from build123d import *

# Parameters (mm, degrees)
SKETCH1_W           = 5
SKETCH1_H           = 54.5
SKETCH1_H_2         = 3
BOSS_EXTRUDE3_DEPTH = 3
SKETCH1_5_W         = 5
SKETCH1_5_H         = 3
BOSS_EXTRUDE4_DEPTH = 11
SKETCH3_W           = 5
SKETCH3_H           = 1
BOSS_EXTRUDE5_DEPTH = 1.5
BOSS_EXTRUDE5_TAPER = 10
BOSS_EXTRUDE6_DEPTH = 5
SKETCH34_W          = 3.5
SKETCH34_H          = 12
BOSS_EXTRUDE2_DEPTH = 12
CUT_EXTRUDE2_REACH  = 46.911
SKETCH4_R           = 2.75


with BuildPart() as part:
    # Sketch1 → Boss-Extrude3 (new body)
    with BuildSketch(Plane.XY):
        with Locations((-78.011372184, 0)):
            Rectangle(SKETCH1_W, SKETCH1_H)
        with Locations((-78.011372184, -28.75)):
            Rectangle(SKETCH1_W, SKETCH1_H_2)
        with Locations((-78.011372184, 28.75)):
            Rectangle(SKETCH1_W, SKETCH1_H_2)
    extrude(amount=BOSS_EXTRUDE3_DEPTH)

    # Sketch1<5> → Boss-Extrude4 (add)
    with BuildSketch(Plane.XY):
        with Locations((-78.011372184, -28.75)):
            Rectangle(SKETCH1_5_W, SKETCH1_5_H)
        with Locations((-78.011372184, 28.75)):
            Rectangle(SKETCH1_5_W, SKETCH1_5_H)
    extrude(amount=-BOSS_EXTRUDE4_DEPTH)

    # Sketch3 → Boss-Extrude5 (add)
    with BuildSketch(Plane(origin=(0, -27.25, 0), x_dir=(1, 0, 0), z_dir=(0, 1, 0))):
        with Locations((-78.011372184, 10.5)):
            Rectangle(SKETCH3_W, SKETCH3_H)
    boss_extrude5 = extrude(amount=BOSS_EXTRUDE5_DEPTH, taper=BOSS_EXTRUDE5_TAPER)

    # Mirror1: Boss-Extrude5 across plane
    add(boss_extrude5.mirror(Plane.ZX))

    # Sketch5 → Boss-Extrude6 (add)
    with BuildSketch(Plane(origin=(-75.511372184, 0, 0), x_dir=(0, 0, -1), z_dir=(1, 0, 0))):
        Polygon((-3, 9.5), (-2, 9.5), (-2, -9.5), (-3, -9.5), (-3, -3.05), (-5.4, -3.05), (-5.4, -5.45), (-6.4, -5.45), (-8, -3.05), (-8, 3.05), (-6.4, 5.45), (-5.4, 5.45), (-5.4, 3.05), (-3, 3.05), align=None)
    extrude(amount=-BOSS_EXTRUDE6_DEPTH)

    # Sketch34 → Boss-Extrude2 (add)
    with BuildSketch(Plane(origin=(-75.511372184, -10.701352109, -2.52337685), x_dir=(0, 0, -1), z_dir=(1, 0, 0))):
        with Locations((-3.77337685, 10.701352109)):
            Rectangle(SKETCH34_W, SKETCH34_H)
    extrude(amount=BOSS_EXTRUDE2_DEPTH)

    # Sketch4 → Cut-Extrude2 (cut, up to next)
    with BuildSketch(Plane(origin=(-75.511372184, -10.701352109, 3), x_dir=(1, 0, 0), z_dir=(0, 0, 1)), mode=Mode.PRIVATE) as cut_extrude2_sk1:
        with Locations((6, 10.701352109)):
            Circle(SKETCH4_R)
    cut_extrude2_tool1 = extrude(cut_extrude2_sk1.sketch, amount=-CUT_EXTRUDE2_REACH, mode=Mode.PRIVATE) & part.part
    add(cut_extrude2_tool1.solids().sort_by_distance((-69.511372, 0, 3))[0], mode=Mode.SUBTRACT)


solid = part.part
The model under review builds one solid part; all positions refer to its coordinate system, in mm. A direction names the side the tool comes from. Coordinates: 2 decimals unless noted, no trailing zeros. Loops run counter-clockwise (first coordinate to the right, second up) from the corner with the lowest first, then second, coordinate; pieces in that order, holes last. Notation, with made-up numbers: (-13, -28) -> (41, -28) arc R9 cw to (41, -19) -> close; hole circle Ø5 at (15, 51.25). An arc over 180 degrees is marked (long way). Use a Markdown table: item, result. Add a question column.
1. Clearance check with flat-ended pins moving along their axes: pin 1 Ø8 at (x, z) = (-68, 0) entering from -Y; pin 2 Ø1.5 at (y, z) = (19.5, 3) entering from +X; pin 3 Ø0.7 at (x, z) = (-77, 4) entering from +Y. State where each tip first meets the part, or that it passes through.
2. Machinability: for faces 1 (the face through (-75.511, 19.9, 0.2)), 2 (the face through (-70, -6, 1)), 3 (the face through (-78, -27.25, -5)), 4 (the face through (-75.511, 0, 6)), which of the approach directions +Z, -Z, +X, -X, +Y, -Y give a long, thin tool a straight path to every point of the face, cutting with its end or side? Answer none if there is none.
3. Add section A-A on y = 0. Write out the cut boundary in (x, z).
4. Add section C-C on x = -68.75. Write out the cut boundary in (y, z), plus the area to 3 significant figures.
5. Draft analysis for pull direction Z (two halves, no side actions). For faces 5 (the face through (-78, -4, 5.4)), 6 (the face through (-78, 29, -11)), 7 (the face through (-70, 6, 1)), state which applies: pulls with the +Z half, pulls with the -Z half, needs draft (parallel to the pull), parting line crosses it, or undercut.
6. To check wall thickness, follow line 1 (Y direction, x = -78, z = -4); line 2 (Z direction, x = -78.75, y = 7); line 3 (Y direction, x = -79, z = 4.75). State the ranges of each line that lie inside material, in increasing order.
7. Add section D-D on z = 2.25. Write out the cut boundary in (x, y), plus the area to 3 significant figures.
8. Add section B-B on z = -3.5. Write out the cut boundary in (x, y), plus the area to 3 significant figures.
Returned:
| question | item | result |
|---|---|---|
| 1 | pin 1 | stops at y = -6 |
| 1 | pin 2 | stops at x = -75.51 |
| 1 | pin 3 | stops at y = 3.05 |
| 2 | face 1 | +Z, -Z, +X, +Y |
| 2 | face 2 | +Z, -Z, +X, -Y |
| 2 | face 3 | +X, -X |
| 2 | face 4 | +Z, +X, +Y, -Y |
| 3 | outline | (-80.51, 0) -> (-75.51, 0) -> (-75.51, -0.5) -> (-72.26, -0.5) -> (-72.26, 3) -> (-75.51, 3) -> (-75.51, 8) -> (-80.51, 8) -> close; (-66.76, -0.5) -> (-63.51, -0.5) -> (-63.51, 3) -> (-66.76, 3) -> close |
| 4 | outline | (-6, -0.5) -> (-2.64, -0.5) -> (-2.64, 3) -> (-6, 3) -> close; (2.64, -0.5) -> (6, -0.5) -> (6, 3) -> (2.64, 3) -> close |
| 4 | area | 23.5 mm² |
| 5 | face 5 | undercut |
| 5 | face 6 | pulls with the -Z half |
| 5 | face 7 | needs draft |
| 6 | line 1 | y = -30.25 to -27.25, 27.25 to 30.25 |
| 6 | line 2 | z = 0 to 3 |
| 6 | line 3 | y = -3.05 to 3.05 |
| 7 | outline | (-80.51, -30.25) -> (-75.51, -30.25) -> (-75.51, -6) -> (-63.51, -6) -> (-63.51, 6) -> (-75.51, 6) -> (-75.51, 30.25) -> (-80.51, 30.25) -> close; hole circle Ø5.5 at (-69.51, 0) |
| 7 | area | 423 mm² |
| 8 | outline | (-80.51, -30.25) -> (-75.51, -30.25) -> (-75.51, -27.25) -> (-80.51, -27.25) -> close; (-80.51, 27.25) -> (-75.51, 27.25) -> (-75.51, 30.25) -> (-80.51, 30.25) -> close |
| 8 | area | 30.0 mm² |
